```python
from build123d import *

# Parameters (mm, degrees)
F0_W      = 101.6
F0_H      = 50.8
F1_DEPTH  = 6.35
F3_DEPTH  = 0.381
F5_DEPTH  = 5.969
F6_R      = 2.54
F7_DEPTH  = 6.35
F8_R      = 2.032
F9_DEPTH  = 5.08
F10_R     = 1.905
F11_DEPTH = 0.381
F12_R     = 0.8001
F13_DEPTH = 0.508


with BuildPart() as f1:
    # F0 (on Top) → F1 (new body)
    with BuildSketch(Plane.XY):
        with Locations((-0.471200794, -2.8610218682)):
            Rectangle(F0_W, F0_H)
    extrude(amount=F1_DEPTH)

    # F2 (on face) → F3 (cut)
    with BuildSketch(Plane(origin=(0, 0, 0), x_dir=(1, 0, 0), z_dir=(0, 0, -1))):
        with BuildLine():
            Line((-38.825200794, -10.0929781318), (-38.825200794, -6.9179781318))
            ThreePointArc((-38.825200794, -6.9179781318), (-41.0702648242, -12.3380421621), (-35.650200794, -10.0929781318))
            Line((-35.650200794, -10.0929781318), (-38.825200794, -10.0929781318))
        make_face()
        with BuildLine():
            Line((37.882799206, -10.0929781318), (37.882799206, -6.9179781318))
            ThreePointArc((37.882799206, -6.9179781318), (35.6377351758, -7.8479141016), (34.707799206, -10.0929781318))
            Line((34.707799206, -10.0929781318), (37.882799206, -10.0929781318))
        make_face()
        with BuildLine():
            ThreePointArc((41.057799206, -10.0929781318), (40.1278632363, -7.8479141016), (37.882799206, -6.9179781318))
            Line((37.882799206, -6.9179781318), (37.882799206, -10.0929781318))
            Line((37.882799206, -10.0929781318), (34.707799206, -10.0929781318))
            ThreePointArc((34.707799206, -10.0929781318), (37.882799206, -13.2679781318), (41.057799206, -10.0929781318))
        make_face()
        with BuildLine():
            Line((34.707799206, 15.8150218682), (-35.650200794, 15.8150218682))
            ThreePointArc((-35.650200794, 15.8150218682), (-36.5801367637, 13.5699578379), (-38.825200794, 12.6400218682))
            Line((-38.825200794, 12.6400218682), (-38.825200794, -6.9179781318))
            ThreePointArc((-38.825200794, -6.9179781318), (-36.5801367637, -7.8479141016), (-35.650200794, -10.0929781318))
            Line((-35.650200794, -10.0929781318), (34.707799206, -10.0929781318))
            ThreePointArc((34.707799206, -10.0929781318), (35.6377351758, -7.8479141016), (37.882799206, -6.9179781318))
            Line((37.882799206, -6.9179781318), (37.882799206, 12.6400218682))
            ThreePointArc((37.882799206, 12.6400218682), (35.6377351758, 13.5699578379), (34.707799206, 15.8150218682))
        make_face()
        with BuildLine():
            ThreePointArc((-35.650200794, -10.0929781318), (-36.5801367637, -7.8479141016), (-38.825200794, -6.9179781318))
            Line((-38.825200794, -6.9179781318), (-38.825200794, -10.0929781318))
            Line((-38.825200794, -10.0929781318), (-35.650200794, -10.0929781318))
        make_face()
        with BuildLine():
            ThreePointArc((41.057799206, 15.8150218682), (37.882799206, 18.9900218682), (34.707799206, 15.8150218682))
            Line((34.707799206, 15.8150218682), (37.882799206, 15.8150218682))
            Line((37.882799206, 15.8150218682), (37.882799206, 12.6400218682))
            ThreePointArc((37.882799206, 12.6400218682), (40.1278632363, 13.5699578379), (41.057799206, 15.8150218682))
        make_face()
        with BuildLine():
            Line((37.882799206, 15.8150218682), (34.707799206, 15.8150218682))
            ThreePointArc((34.707799206, 15.8150218682), (35.6377351758, 13.5699578379), (37.882799206, 12.6400218682))
            Line((37.882799206, 12.6400218682), (37.882799206, 15.8150218682))
        make_face()
        with BuildLine():
            Line((-35.650200794, 15.8150218682), (-38.825200794, 15.8150218682))
            Line((-38.825200794, 15.8150218682), (-38.825200794, 12.6400218682))
            ThreePointArc((-38.825200794, 12.6400218682), (-36.5801367637, 13.5699578379), (-35.650200794, 15.8150218682))
        make_face()
        with BuildLine():
            Line((-38.825200794, 12.6400218682), (-38.825200794, 15.8150218682))
            Line((-38.825200794, 15.8150218682), (-35.650200794, 15.8150218682))
            ThreePointArc((-35.650200794, 15.8150218682), (-41.0702648242, 18.0600858984), (-38.825200794, 12.6400218682))
        make_face()
    extrude(amount=-F3_DEPTH, mode=Mode.SUBTRACT)

    # F4 (on face) → F5 (cut, through all)
    with BuildSketch(Plane(origin=(0, 0, 0.381), x_dir=(1, 0, 0), z_dir=(0, 0, -1))):
        with BuildLine():
            Line((14.768799206, 13.0210218682), (2.068799206, 13.0210218682))
            ThreePointArc((2.068799206, 13.0210218682), (0.2727479818, 12.2770730924), (-0.471200794, 10.4810218682))
            Line((-0.471200794, 10.4810218682), (-0.471200794, -4.7589781318))
            ThreePointArc((-0.471200794, -4.7589781318), (0.2727479818, -6.555029356), (2.068799206, -7.2989781318))
            Line((2.068799206, -7.2989781318), (14.768799206, -7.2989781318))
            ThreePointArc((14.768799206, -7.2989781318), (16.5648504302, -6.555029356), (17.308799206, -4.7589781318))
            Line((17.308799206, -4.7589781318), (17.308799206, 10.4810218682))
            ThreePointArc((17.308799206, 10.4810218682), (16.5648504302, 12.2770730924), (14.768799206, 13.0210218682))
        make_face()
    extrude(amount=-F5_DEPTH, mode=Mode.SUBTRACT)

    # F6 (on face) → F7 (cut, through all)
    with BuildSketch(Plane(origin=(0, 0, 0), x_dir=(1, 0, 0), z_dir=(0, 0, -1))):
        with Locations((-44.921200794, 21.9110218682)):
            Circle(F6_R)
        with Locations((43.978799206, 21.9110218682)):
            Circle(F6_R)
        with Locations((43.978799206, -16.1889781318)):
            Circle(F6_R)
        with Locations((-0.471200794, -16.1889781318)):
            Circle(F6_R)
        with Locations((-44.921200794, -16.1889781318)):
            Circle(F6_R)
        with Locations((-0.471200794, 21.9110218682)):
            Circle(F6_R)
    extrude(amount=-F7_DEPTH, mode=Mode.SUBTRACT)

    # F8 (on face) → F9 (cut)
    with BuildSketch(Plane.XY.offset(6.35)):
        with Locations((-22.371080794, -2.8610218682)):
            Circle(F8_R)
        with Locations((-11.972320794, -2.8610218682)):
            Circle(F8_R)
        with Locations((-3.971320794, 3.6388381318)):
            Circle(F8_R)
        with Locations((-3.971320794, -9.3608818682)):
            Circle(F8_R)
        with Locations((21.428679206, -2.8610218682)):
            Circle(F8_R)
    extrude(amount=-F9_DEPTH, mode=Mode.SUBTRACT)

    # F10 (on face) → F11 (cut)
    with BuildSketch(Plane(origin=(0, 0, 0.381), x_dir=(1, 0, 0), z_dir=(0, 0, -1))):
        with Locations((-22.366000794, 2.8610218682)):
            Circle(F10_R)
        with Locations((-11.977400794, 2.8610218682)):
            Circle(F10_R)
        with Locations((-3.976400794, 9.3634218682)):
            Circle(F10_R)
        with Locations((-3.976400794, -3.6413781318)):
            Circle(F10_R)
        with Locations((21.423599206, 2.8610218682)):
            Circle(F10_R)
    extrude(amount=-F11_DEPTH, mode=Mode.SUBTRACT)

    # F12 (on face) → F13 (cut, through all)
    with BuildSketch(Plane(origin=(0, 0, 0.762), x_dir=(1, 0, 0), z_dir=(0, 0, -1))):
        with Locations((-22.366000794, 2.8610218682)):
            Circle(F12_R)
        with Locations((-11.977400794, 2.8610218682)):
            Circle(F12_R)
        with Locations((-3.976400794, 9.3634218682)):
            Circle(F12_R)
        with Locations((-3.976400794, -3.6413781318)):
            Circle(F12_R)
        with Locations((21.423599206, 2.8610218682)):
            Circle(F12_R)
    extrude(amount=-F13_DEPTH, mode=Mode.SUBTRACT)


solid = f1.part
```
Check sheet for the modelled part. Datum: model origin and axes. Units: mm. A direction names the side the tool comes from. Round coordinates to 2 decimals unless told otherwise and drop trailing zeros. Order: outer loops, then holes, each group sorted by start corner. A loop starts at its lowest first (then second) coordinate and runs counter-clockwise, first axis right, second up. Notation, with made-up numbers: M -32,-17 L -13,-17 A33 cw -13,17 Z; hole C 71.5,49 d1. An arc over 180 degrees is marked long. Answer in a Markdown table with one row per item.
(1) Gauge pin test, flat ends, axial feed: pin 1 (3.5 mm diameter, centred on x = -22.5, y = -2, fed in from +Z); pin 2 (4 mm diameter, centred on x = -7.5, y = 6, fed in from -Z); pin 3 (1.1 mm diameter, centred on x = 21, y = -2.5, fed in from -Z); pin 4 (3 mm diameter, centred on x = -11.98, y = -2.86, fed in from +Z). Record the tip position at first contact, or that the pin passes through.
Findings:
| item | result |
|---|---|
| pin 1 | stops at z = 6.35 |
| pin 2 | stops at z = 0.38 |
| pin 3 | stops at z = 0.76 |
| pin 4 | stops at z = 1.27 |
(2) Section check B-B on x = 43.5. Record the boundary of the cut face in (y, z), plus the area to 3 significant figures.
Findings:
| item | result |
|---|---|
| outline | M -28.26,0 L -24.41,0 L -24.41,6.35 L -28.26,6.35 Z; M -19.42,0 L 13.69,0 L 13.69,6.35 L -19.42,6.35 Z; M 18.68,0 L 22.54,0 L 22.54,6.35 L 18.68,6.35 Z |
| area | 259 mm^2 |
(3) Section check C-C on z = 4.25. Give the number of separate pieces and of enclosed holes in the cut face, plus the area to 3 significant figures.
Findings:
| item | result |
|---|---|
| separate pieces | 1 |
| enclosed holes | 12 |
| area | 4,620 mm^2 |
(4) Section check A-A on x = 26.5. Record the boundary of the cut face in (y, z).
Findings:
| item | result |
|---|---|
| outline | M -28.26,0 L -15.82,0 L -15.82,0.38 L 10.09,0.38 L 10.09,0 L 22.54,0 L 22.54,6.35 L -28.26,6.35 Z |
(5) Set-up check for faces 1 (the cylindrical face through (19.4, -2.77, 3.85)), 2 (the cylindrical face through (16.58, -12.26, 3.32)), 3 (the cylindrical face through (-20.606, -2.131, 0.569)): record each of +Z, -Z, +X, -X, +Y, -Y from which the full face is reachable in a straight line by a thin tool's end or side.
Findings:
| item | result |
|---|---|
| face 1 | +Z |
| face 2 | +Z, -Z |
| face 3 | -Z |
(6) Material ranges on line 1 along X through (y, z) = (-3, 2); line 2 along X through (y, z) = (-9.5, 4.75); line 3 along Y through (x, z) = (-44, 5.5), recorded low to high. Write a range as from..to.
Findings:
| item | result |
|---|---|
| line 1 | x = -51.27..-24.4, -20.34..-14, -9.95..-0.47, 17.31..19.4, 23.46..50.33 |
| line 2 | x = -51.27..-6, -1.94..-0.47, 17.31..50.33 |
| line 3 | y = -28.26..-24.28, -19.54..13.82, 18.56..22.54 |
(7) Draft check along X on faces 4 (the flat face through (-1, 22.539, 3)), 5 (the flat face through (-1, -3, 0.381)), 6 (the flat face through (50.329, -3, 3)). Enter one of: +X half, -X half, draft (parallel to the pull), parting line (faces both ways), or undercut.
Findings:
| item | result |
|---|---|
| face 4 | draft |
| face 5 | undercut |
| face 6 | +X half |
(8) Section check D-D on y = -14.5. Record the boundary of the cut face in (x, z).
Findings:
| item | result |
|---|---|
| outline | M -51.27,0 L -41.72,0 L -41.72,0.38 L 40.77,0.38 L 40.77,0 L 50.33,0 L 50.33,6.35 L -51.27,6.35 Z |
